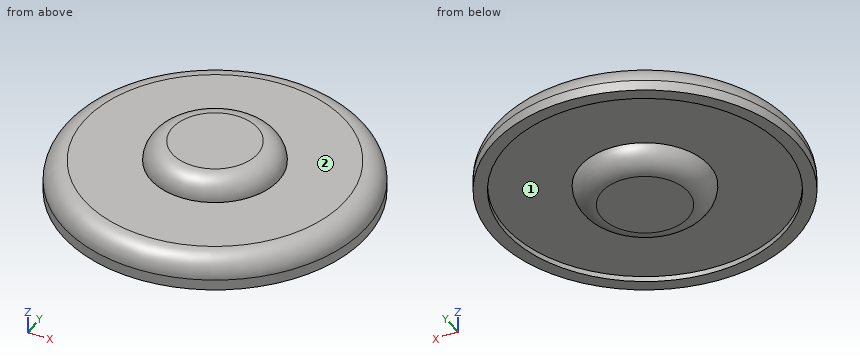
Autodesk Inventor part; units mm, degrees
ref_plane "YZ Plane" through (0, 0, 0) normal (1, 0, 0) x (0, 1, 0)
ref_plane "XZ Plane" through (0, 0, 0) normal (0, 1, 0) x (-1, 0, 0)
ref_plane "XY Plane" through (0, 0, 0) normal (0, 0, 1) x (1, 0, 0)
sketch "Sketch1" plane through (0, 0, 0) normal (0, 0, 1) x (1, 0, 0)
  circle A0 centre (0, 0) radius 14.25
  dimension "d0" = 28.5
extrude "Extrusion1" add sketch "Sketch1" along normal blind 3
sketch "Sketch2" plane through (0, 0, 3) normal (0, 0, 1) x (1, 0, 0)
  circle A0 centre (0, 0) radius 6
  dimension "d3" = 12
extrude "Extrusion2" add sketch "Sketch2" along normal blind 2
fillet "Fillet1" radius 2 1 edges at (-14.25, 0, 3)
fillet "Fillet2" radius 2 1 edges at (-6, 0, 5)
sketch "Sketch3" plane through (0, 0, 0) normal (0, 0, -1) x (-1, 0, 0)
  circle A0 centre (0, 0) radius 13.0539
extrude "Extrusion3" cut sketch "Sketch3" against normal blind 0.5
sketch "Sketch4" plane through (0, 0, 0.5) normal (0, 0, -1) x (-1, 0, 0)
  circle A0 centre (0, 0) radius 6.0392
extrude "Extrusion4" add sketch "Sketch4" along normal blind 2
fillet "Fillet3" radius 2 1 edges at (6.0392, 0, -1.5)
properties part number "speaker"
Read the model definition and answer for the solid it produces. Units are mm, in the model's axes. Face numbers are marked on the shaded views. Coordinates: 2 decimals unless noted, no trailing zeros. Write each loop counter-clockwise with the first axis right and the second up, starting at its lowest first coordinate (ties: lowest second). Pieces come first, ordered by that corner, then holes. Notation, with made-up numbers: (-1, -23) -> (43, -23) arc R16 ccw to (43, -15) -> close; hole circle Ø7 at (57, 47.5). An arc over 180 degrees is marked (long way). Return JSON: item names as keys, results as strings.
(1) For a pull along X with two mould halves and no side action, classify the marked faces 1 and 2 as pulls with the +X half, pulls with the -X half, needs draft (parallel to the pull), parting line crosses it, or undercut.
Answers below:
{"face 1": "undercut", "face 2": "needs draft"}
(2) The part is cut by section C-C on z = 3.75. Give the vertices of the cut face in (x, y).
Answers below:
{"outline": "circle Ø11.71 at (0, 0)"}
(3) Each of these flat-tipped pins is pushed along its axis until it touches: P1, Ø10, axis at x = 3.5, y = -4.5, coming from the -Z side; P2, Ø2, axis at y = -1.5, z = 4.5, coming from the +X side; P3, Ø4, axis at x = -8.5, y = -10.5, coming from the +Z side. Where does it stop, or does it pass through?
Answers below:
{"P1": "z = -1.5", "P2": "x = 5.81", "P3": "z = 3"}
(4) Consider line 1 along Y through (x, z) = (0, 0.3); line 2 along Z through (x, y) = (-8.75, 4.5); line 3 along Z through (x, y) = (-11.5, -7.25). Determine where each line is inside the solid, lowest interval first. Write a range as from..to.
Answers below:
{"line 1": "-14.25..-13.05, -6.03..6.03, 13.05..14.25", "line 2": "0.5..3", "line 3": "0..2.48"}
